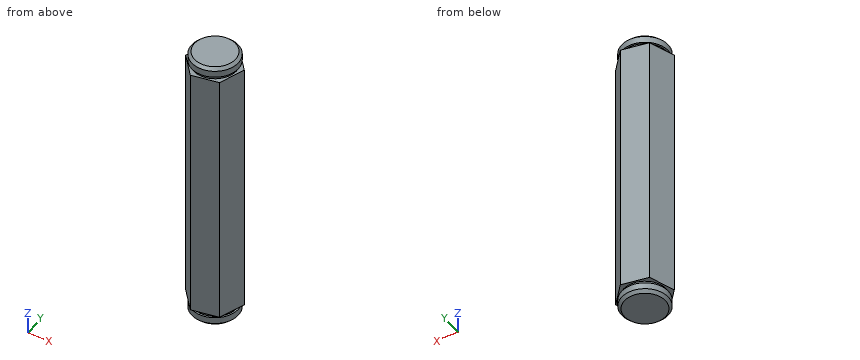
```python
from build123d import *

# Parameters (mm, degrees)
BOSS_EXTRUDE1_DEPTH      = 35.56
SKETCH2_R                = 5.8547
BOSS_EXTRUDE2_DEPTH      = 0.889
SKETCH3_R                = 6.35
BOSS_EXTRUDE3_DEPTH      = 2.54
CHAMFER1_SIZE            = 0.762
CHAMFER1_OF_MIRROR1_SIZE = 0.762


with BuildPart() as part:
    # Sketch1 → Boss-Extrude1 (new, symmetric)
    with BuildSketch(Plane.XY):
        Polygon((-2.440353064, -6.914333681), (4.767812086, -5.570574588), (7.20816515, 1.343759093), (2.440353064, 6.914333681), (-4.767812086, 5.570574588), (-7.20816515, -1.343759093), align=None)
    extrude(amount=BOSS_EXTRUDE1_DEPTH, both=True)

    # Sketch2 → Boss-Extrude2 (add)
    with BuildSketch(Plane.XY.offset(35.56)):
        Circle(SKETCH2_R)
    boss_extrude2 = extrude(amount=BOSS_EXTRUDE2_DEPTH)

    # Sketch3 → Boss-Extrude3 (add)
    with BuildSketch(Plane.XY.offset(36.449)):
        Circle(SKETCH3_R)
    boss_extrude3 = extrude(amount=BOSS_EXTRUDE3_DEPTH)

    # Chamfer1
    chamfer1_edges = [part.edges().sort_by_distance(p)[0] for p in [
        (-6.35, 0, 38.989),
    ]]
    chamfer(chamfer1_edges, length=CHAMFER1_SIZE)

    # Mirror1: Boss-Extrude2, Boss-Extrude3 across plane
    add(boss_extrude2.mirror(Plane.XY))
    add(boss_extrude3.mirror(Plane.XY))

    # Chamfer1 of Mirror1
    chamfer1_of_mirror1_edges = [part.edges().sort_by_distance(p)[0] for p in [
        (-6.35, 0, -38.989),
    ]]
    chamfer(chamfer1_of_mirror1_edges, length=CHAMFER1_OF_MIRROR1_SIZE)


solid = part.part
```
Geometry: final body of the model. Coordinates: model frame, mm. Give positions to 0.01 mm unless a question says otherwise; leave off trailing zeros. Order: outer loops, then holes, each group sorted by start corner. A loop starts at its lowest first (then second) coordinate and runs counter-clockwise, first axis right, second up. Notation, with made-up numbers: (-8.5, 36) -> (48.5, 36) arc R23 cw to (48.5, 63) -> close; hole circle Ø9 at (82.5, -17). An arc over 180 degrees is marked (long way). Write each question's results on one line, items separated by ' | '. Start each with the question number.
1) First-contact query: pin 1 (1 mm diameter, centred on x = 1.5, y = -5.5, fed in from -Z); pin 2 (3 mm diameter, centred on y = 0.5, z = 17, fed in from -X); pin 3 (2 mm diameter, centred on x = 2.5, z = -1.5, fed in from -Y). Flat tips, straight axial feed; report the tip coordinate or a pass-through.
2) Section B-B (y = 0). Return loops of the section in (x, z), then the cut area to 3 significant figures.
3) Line query: line 1 (Z direction, x = -5, y = 3.5); line 2 (Z direction, x = 4, y = -4.5); line 3 (X direction, y = 5, z = -29). Output: solid intervals per line, ascending. Write a range as from..to.
4) Section A-A (z = 14.5). Return loops of the section in (x, y).
5) Section C-C (x = 0). Return loops of the section in (y, z), then the cut area to 3 significant figures.
Calculated:
1) pin 1: z = -38.99 | pin 2: x = -7.09 | pin 3: y = -6.18
2) outline: (-6.73, -35.56) -> (-5.85, -35.56) -> (-5.85, -36.45) -> (-6.35, -36.45) -> (-6.35, -38.23) -> (-5.59, -38.99) -> (5.59, -38.99) -> (6.35, -38.23) -> (6.35, -36.45) -> (5.85, -36.45) -> (5.85, -35.56) -> (6.73, -35.56) -> (6.73, 35.56) -> (5.85, 35.56) -> (5.85, 36.45) -> (6.35, 36.45) -> (6.35, 38.23) -> (5.59, 38.99) -> (-5.59, 38.99) -> (-6.35, 38.23) -> (-6.35, 36.45) -> (-5.85, 36.45) -> (-5.85, 35.56) -> (-6.73, 35.56) -> close | area: 1,040 mm2
3) line 1: -38.47..-36.45, -35.56..35.56, 36.45..38.47 | line 2: -38.56..-36.45, -35.56..35.56, 36.45..38.56 | line 3: -4.97..4.08
4) outline: (-7.21, -1.34) -> (-2.44, -6.91) -> (4.77, -5.57) -> (7.21, 1.34) -> (2.44, 6.91) -> (-4.77, 5.57) -> close
5) outline: (-6.46, -35.56) -> (-5.85, -35.56) -> (-5.85, -36.45) -> (-6.35, -36.45) -> (-6.35, -38.23) -> (-5.59, -38.99) -> (5.59, -38.99) -> (6.35, -38.23) -> (6.35, -36.45) -> (5.85, -36.45) -> (5.85, -35.56) -> (6.46, -35.56) -> (6.46, 35.56) -> (5.85, 35.56) -> (5.85, 36.45) -> (6.35, 36.45) -> (6.35, 38.23) -> (5.59, 38.99) -> (-5.59, 38.99) -> (-6.35, 38.23) -> (-6.35, 36.45) -> (-5.85, 36.45) -> (-5.85, 35.56) -> (-6.46, 35.56) -> close | area: 1,000 mm2
